from build123d import *

# Parameters (mm, degrees)
BOSS_EXTRUDE1_DEPTH         = 6.35
BOSS_EXTRUDE3_DEPTH         = 6.35
F_1_4_CLEARANCE_HOLE1_D     = 6.7564
TAP_DRILL_FOR_1_4_20_TAP1_D = 5.08
BOSS_EXTRUDE4_DEPTH         = 6.35


with BuildPart() as part:
    # Sketch2 → Boss-Extrude1 (new body)
    with BuildSketch(Plane(origin=(0, 0, 0), x_dir=(1, 0, 0), z_dir=(0, 1, 0))):
        Polygon((2.766393585, 15.625659676), (9.035920728, -1.599724579), (3.144492336, -8.62085553), (-14.907891591, -5.437733178), (-33.036934837, 9.774340324), (-39.306461979, 26.999724579), (-33.415033588, 34.02085553), (-15.362649661, 30.837733178), align=None)
    extrude(amount=-BOSS_EXTRUDE1_DEPTH)

    # Sketch7 → Boss-Extrude3 (add)
    with BuildSketch(Plane.XZ.offset(6.35)):
        Polygon((2.766393585, -15.625659676), (11.284005931, -25.77655479), (11.284005931, -208.646188628), (2.766393585, -218.797083741), (9.035920728, -236.022467996), (3.144492336, -243.043598948), (-14.907891591, -239.860476595), (-33.036934837, -224.648403094), (-39.306461979, -207.423018839), (-33.415033588, -200.401887887), (-15.362649661, -203.58501024), (-12.381779272, -200.032547244), (-12.381779272, -34.390196174), (-15.362649661, -30.837733178), align=None)
    extrude(amount=-BOSS_EXTRUDE3_DEPTH)

    # 1/4 Clearance Hole1 (through all)
    with Locations(Plane(origin=(0, 0, 0), x_dir=(1, 0, 0), z_dir=(0, 1, 0))):
        with Locations((0, 0), (3.333805931, 77.211371709), (3.333805931, 157.211371709), (0, 234.422743417)):
            Hole(F_1_4_CLEARANCE_HOLE1_D / 2)

    # Tap Drill for 1/4-20 Tap1 (through all)
    with Locations(Plane(origin=(0, 0, 0), x_dir=(1, 0, 0), z_dir=(0, 1, 0))):
        with Locations((-14.247913361, 8.043291), (-14.247913361, 226.379452417)):
            Hole(TAP_DRILL_FOR_1_4_20_TAP1_D / 2)

    # Sketch10 → Boss-Extrude4 (add)
    with BuildSketch(Plane.XZ.offset(6.35)):
        Polygon((-14.907891591, -239.860476595), (-23.425503936, -250.011371709), (-39.306461979, -250.011371709), (-39.306461979, -207.423018839), (-33.036934837, -224.648403094), align=None)
        Polygon((-14.907891591, 5.437733178), (-23.425503936, 15.588628291), (-39.306461979, 15.588628291), (-39.306461979, -26.999724579), (-33.036934837, -9.774340324), align=None)
    extrude(amount=-BOSS_EXTRUDE4_DEPTH)


solid = part.part
CAD build for the part. Positions are in the model's coordinates, mm. A direction names the side the tool comes from. Round coordinates to 2 decimals unless told otherwise and drop trailing zeros. Write each loop counter-clockwise with the first axis right and the second up, starting at its lowest first coordinate (ties: lowest second). Pieces come first, ordered by that corner, then holes. Notation, with made-up numbers: M 89.5,-9.75 L 143.5,-9.75 A4 cw 143.5,-5.75 Z; hole C -39,-22.5 d2. An arc over 180 degrees is marked long. Use a Markdown table: item, result. Add a question column.
1. Flat gauge pins, fed straight in: P1, Ø2, axis at x = -22, y = -5, coming from the -Z side; P2, Ø2, axis at x = -5, y = -4, coming from the +Z side. Where does each tip first touch, or does it go through?
2. Pull direction Z, two halves, no side cores. Call faces 6 (the face through (11.284, -3, -116)), 7 (the face through (4.066, -3.219, -153.914)), 8 (the face through (-31, -3, 15.589)): released by +Z, released by -Z, zero draft, split by the parting line, or undercut.
3. Drill centre lines: probe 1 along Z at (x, y) = (-16.5, -0.25); probe 2 along Z at (x, y) = (-14.5, -5.5); probe 3 along Z at (x, y) = (-17.5, -1.75). Where is each one in solid material? Low to high.
4. Slice it at C-C on z = -97. Give the cut face in (x, y).
5. Slice it at A-A on x = -21. Give the cut face in (y, z).
6. 3-axis set-ups, long thin cutter, end or side, ignore diameter. For faces 1 (the face through (-12.382, -3, -118)), 2 (the face through (-24.52, -3.22, -201.97)), 3 (the face through (-5.76, -3.13, 7.05)), 4 (the face through (7.085, -3.219, -213.651)), 5 (the face through (-5.755, -3.219, -241.474)): which of +Z, -Z, +X, -X, +Y, -Y reach the whole face in a straight line?
7. Slice it at B-B on y = -5. Give the cut face in (x, z), then the cut area to 3 significant figures.
Reply:
| question | item | result |
|---|---|---|
| 1 | P1 | stops at z = -249.5 |
| 1 | P2 | stops at z = 7.36 |
| 2 | face 6 | zero draft |
| 2 | face 7 | undercut |
| 2 | face 8 | released by +Z |
| 3 | probe 1 | z = -241.76 to -227.55, -225.2 to -203.38, -31.04 to -9.22, -6.87 to 7.34 |
| 3 | probe 2 | z = -239.93 to -228.91, -223.85 to -202.56, -31.87 to -10.57, -5.52 to 5.51 |
| 3 | probe 3 | z = -242.95 to -203.21, -31.21 to 8.53 |
| 4 | outline | M -12.38,-6.35 L 11.28,-6.35 L 11.28,0 L -12.38,0 Z |
| 5 | outline | M -6.35,-247.12 L 0,-247.12 L 0,-202.59 L -6.35,-202.59 Z; M -6.35,-31.83 L 0,-31.83 L 0,12.7 L -6.35,12.7 Z |
| 6 | face 1 | -X, +Y, -Y |
| 6 | face 2 | +Y, -Y |
| 6 | face 3 | +Z, +Y, -Y |
| 6 | face 4 | +X, +Y, -Y |
| 6 | face 5 | -Z, +Y, -Y |
| 7 | outline | M -39.31,-250.01 L -23.43,-250.01 L -14.91,-239.86 L 3.14,-243.04 L 9.04,-236.02 L 2.77,-218.8 L 11.28,-208.65 L 11.28,-25.78 L 2.77,-15.63 L 9.04,1.6 L 3.14,8.62 L -14.91,5.44 L -23.43,15.59 L -39.31,15.59 L -39.31,-27 L -33.42,-34.02 L -15.36,-30.84 L -12.38,-34.39 L -12.38,-200.03 L -15.36,-203.59 L -33.42,-200.4 L -39.31,-207.42 Z; hole C -14.25,-226.38 d5.08; hole C -14.25,-8.04 d5.08; hole C 0,-234.42 d6.76; hole C 0,0 d6.76; hole C 3.33,-157.21 d6.76; hole C 3.33,-77.21 d6.76 |
| 7 | area | 7,810 mm^2 |
